```python
from build123d import *

# Parameters (mm, degrees)
F1_DEPTH = 11.1125
F2_R     = 7.9375
F3_DEPTH = 133.096
F5_DEPTH = 135.636
F6_W     = 2.54
F6_H     = 2.54
F7_DEPTH = 3.81
F8_W     = 2.032
F8_H     = 2.032
F9_DEPTH = 2.54


with BuildPart() as f1:
    # F0 (on Front) → F1 (new body, symmetric)
    with BuildSketch(Plane.XZ):
        Polygon((-11.1125, -58.42), (11.1125, -58.42), (11.1125, -35.3219639331), (0, -46.4344639331), (0, -29.8688001931), (11.1125, -20.1350393977), (11.1125, 58.42), (-11.1125, 58.42), (-11.1125, 25.0589007236), (0, 17.3320677131), (0, -1.5664904641), (-11.1125, 7.9825179157), align=None)
        Polygon((0, -46.4344639331), (11.1125, -35.3219639331), (11.1125, -20.1350393977), (0, -29.8688001931), align=None)
        Polygon((11.1125, -20.1350393977), (11.1125, -35.3219639331), (59.3725, 12.9380360669), (54.7055751085, 18.0493984371), (30.8782853477, -2.8216151901), (24.0951018289, -8.763202214), align=None)
        Polygon((-59.3725, 49.452497165), (-11.1125, 7.9825179157), (-11.1125, 25.0589007236), (-54.0828680275, 54.9374031437), align=None)
        Polygon((-11.1125, 25.0589007236), (-11.1125, 7.9825179157), (0, -1.5664904641), (0, 17.3320677131), align=None)
        Polygon((24.4025364518, 13.2276853547), (24.0951018289, -8.763202214), (30.8782853477, -2.8216151901), (29.1275199493, 13.2276853547), align=None)
    extrude(amount=F1_DEPTH, both=True)

    # F2 (on face) → F3 (cut)
    with BuildSketch(Plane.XY.offset(58.42)):
        Circle(F2_R)
    extrude(amount=-F3_DEPTH, mode=Mode.SUBTRACT)

    # F4 (on face) → F5 (cut)
    with BuildSketch(Plane.XY.offset(58.42)):
        Polygon((-61.5530486068, -11.1125), (-11.1125, -11.1125), (-61.5530486068, -5.08), align=None)
        Polygon((-61.5530486068, 5.08), (-11.1125, 11.1125), (-61.5530486068, 11.1125), align=None)
        Polygon((61.5530486068, -5.08), (11.1125, -11.1125), (61.5530486068, -11.1125), align=None)
        Polygon((61.5530486068, 11.1125), (11.1125, 11.1125), (61.5530486068, 5.08), align=None)
    extrude(amount=-F5_DEPTH, mode=Mode.SUBTRACT)

    # F6 (on face) → F7 (cut)
    with BuildSketch(Plane(origin=(0, 0, -58.42), x_dir=(1, 0, 0), z_dir=(0, 0, -1))):
        with Locations((8.5725, 8.5725)):
            Rectangle(F6_W, F6_H)
        with Locations((-8.5725, -8.5725)):
            Rectangle(F6_W, F6_H)
    extrude(amount=-F7_DEPTH, mode=Mode.SUBTRACT)

    # F8 (on face) → F9 (join)
    with BuildSketch(Plane.XY.offset(58.42)):
        with Locations((8.5725, -8.5725)):
            Rectangle(F8_W, F8_H)
        with Locations((-8.5725, 8.5725)):
            Rectangle(F8_W, F8_H)
    extrude(amount=F9_DEPTH)


solid = f1.part
```
Input: part model. Units: mm. Frame: model coordinates. A direction names the side the tool comes from. Round coordinates to 2 decimals unless told otherwise and drop trailing zeros. Write each loop counter-clockwise with the first axis right and the second up, starting at its lowest first coordinate (ties: lowest second). Pieces come first, ordered by that corner, then holes. Notation, with made-up numbers: (-25, 80) -> (-1, 80) arc R9 ccw to (-1, 91) -> close; hole circle Ø5 at (13.5, 3.25). An arc over 180 degrees is marked (long way). Answer as CSV lines item,"result".
1. Section A-A (y = 0). Return the cut outline in (x, z).
Geometry says:
outline,"(-59.37, 49.45) -> (-11.11, 7.98) -> (-11.11, -58.42) -> (-7.94, -58.42) -> (-7.94, 58.42) -> (-11.11, 58.42) -> (-11.11, 25.06) -> (-54.08, 54.94) -> close; (7.94, -58.42) -> (11.11, -58.42) -> (11.11, -35.32) -> (59.37, 12.94) -> (54.71, 18.05) -> (30.88, -2.82) -> (29.13, 13.23) -> (24.4, 13.23) -> (24.1, -8.76) -> (11.11, -20.14) -> (11.11, 58.42) -> (7.94, 58.42) -> close"
2. Reachability of faces 4 (the flat face through (11.112, 0, -47)), 5 (the flat face through (-32.3, -0.16, 39.79)), 6 (the flat face through (31.78, -8.64, -4.56)), 7 (the flat face through (-11.112, 0, -25)) from +Z, -Z, +X, -X, +Y, -Y: full face, straight path, thin tool, end or side. Return the list, or none.
Geometry says:
face 4,"-Z, +X, +Y, -Y"
face 5,"+Z, +Y, -Y"
face 6,"+Z, -Z, +X, -Y"
face 7,"-Z, -X, +Y, -Y"
3. Section D-D (z = -39). Return the cut outline in (x, y) (1 decimal), plus the area to 3 significant figures.
Geometry says:
outline,"(-11.1, -11.1) -> (11.1, -11.1) -> (11.1, 11.1) -> (-11.1, 11.1) -> close; hole circle Ø15.9 at (0, 0)"
area,"296 mm^2"
4. Section B-B (x = 0). Return the cut outline in (y, z), plus the area to 3 significant figures.
Geometry says:
outline,"(-11.11, -58.42) -> (-7.94, -58.42) -> (-7.94, 58.42) -> (-11.11, 58.42) -> close; (7.94, -58.42) -> (11.11, -58.42) -> (11.11, 58.42) -> (7.94, 58.42) -> close"
area,"742 mm^2"
5. Contact query for flat-ended pins moving along their axis: P1, Ø8, axis at x = -34.5, y = 7.5, coming from the +Z side; P2, Ø1.6, axis at y = 8.5, z = 59.5, coming from the -X side; P3, Ø2, axis at y = -2, z = 19, coming from the -X side. Output: stop coordinate, or through.
Geometry says:
P1,"stops at z = 44.1"
P2,"stops at x = -9.59"
P3,"stops at x = -25.1"
6. Section C-C (z = 2). Return the cut outline in (x, y) (1 decimal), plus the area to 3 significant figures.
Geometry says:
outline,"(-11.1, -11.1) -> (11.1, -11.1) -> (11.1, 11.1) -> (-11.1, 11.1) -> close; (24.2, -9.5) -> (30.4, -8.8) -> (30.4, 8.8) -> (24.2, 9.5) -> close; (36.4, -8.1) -> (48.4, -6.6) -> (48.4, 6.6) -> (36.4, 8.1) -> close; hole circle Ø15.9 at (0, 0)"
area,"586 mm^2"
7. Ray query, L1, parallel to X at y = 4.5, z = 15.5; L2, parallel to X at y = 4, z = -9.5; L3, parallel to Y at x = 0, z = 32. Return the intervals inside material, ascending. Write a range as [from, to].
Geometry says:
L1,"x = [-19.86, -6.54], [6.54, 11.11], [51.8, 57.03]"
L2,"x = [-11.11, -6.86], [6.86, 11.11], [23.25, 36.93]"
L3,"y = [-11.11, -7.94], [7.94, 11.11]"
8. Mould query, pull axis Y, two halves, no side actions, for faces 1 (the cylindrical face through (-1.72, -7.75, 0.82)), 2 (the flat face through (57.07, -0.08, 15.46)), 3 (the flat face through (-31.555, -8.668, 31.57)). Classes: +Y half, -Y half, draft (parallel to the pull), parting line (faces both ways), or undercut.
Geometry says:
face 1,"undercut"
face 2,"draft"
face 3,"-Y half"
